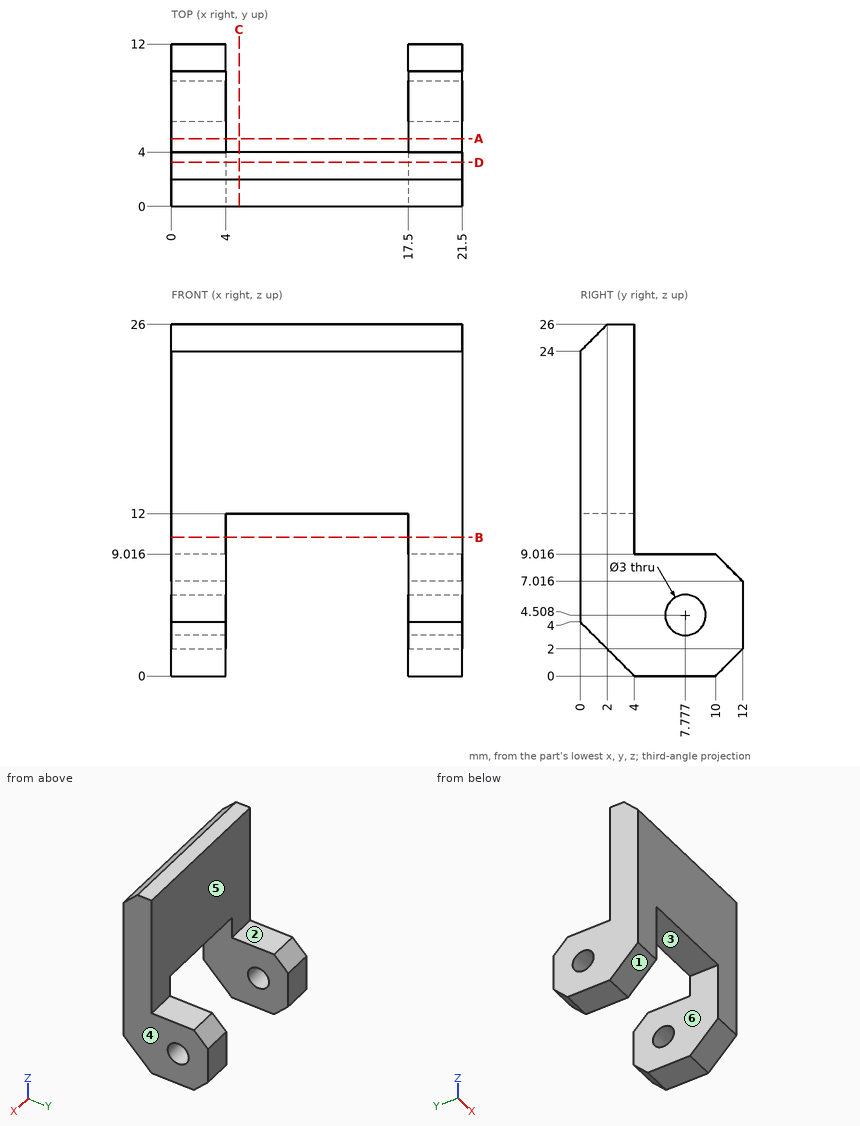
Check sheet for the drawn part. Datum: minimum x, y, z corner. Units: mm. A direction names the side the tool comes from. Round coordinates to 2 decimals unless told otherwise and drop trailing zeros. Write each loop counter-clockwise with the first axis right and the second up, starting at its lowest first coordinate (ties: lowest second). Pieces come first, ordered by that corner, then holes. Notation, with made-up numbers: (33, 5) -> (88, 5) arc R11 cw to (88, 9) -> close; hole circle Ø2 at (-33, 85.25). An arc over 180 degrees is marked (long way). Write each question's results on one line, items separated by ' | '. Start each with the question number.
1. Cross-section at C-C (x = 5). Enter the section's corners in (y, z).
2. Set-up check for the marked faces 1 and 2: record each of +Z, -Z, +X, -X, +Y, -Y from which the full face is reachable in a straight line by a thin tool's end or side.
3. Cross-section at B-B (z = 10.25). Enter the section's corners in (x, y).
4. Cross-section at A-A (y = 5). Enter the section's corners in (x, z).
5. Draft check along X on the marked faces 3, 4, 5 and 6. Enter one of: +X half, -X half, draft (parallel to the pull), parting line (faces both ways), or undercut.
6. Cross-section at D-D (y = 3.25). Enter the section's corners in (x, z).
7. Material ranges on probe 1 along X at (y, z) = (8.75, 3); probe 2 along Y at (x, z) = (8.25, 18.25); probe 3 along Z at (x, y) = (13, 2.75), recorded low to high. Write a range as from..to.
8. Depth check by flat-ended pin: P1, Ø5, axis at y = 4.5, z = 14, coming from the +X side; P2, Ø3, axis at x = 14, y = 3, coming from the -Z side; P3, Ø2, axis at x = 19, y = 8, coming from the +Z side; P4, Ø8.5, axis at x = 9, z = 16.5, coming from the +Y side. Enter the tip coordinate at first touch or a pass-through.
Solutions:
1) outline: (0, 12) -> (4, 12) -> (4, 26) -> (2, 26) -> (0, 24) -> close
2) face 1: -Z, +X, -X, -Y | face 2: +Z, +X, -X, +Y
3) outline: (0, 0) -> (4, 0) -> (4, 4) -> (0, 4) -> close; (17.5, 0) -> (21.5, 0) -> (21.5, 4) -> (17.5, 4) -> close
4) outline: (0, 0) -> (4, 0) -> (4, 9.02) -> (0, 9.02) -> close; (17.5, 0) -> (21.5, 0) -> (21.5, 9.02) -> (17.5, 9.02) -> close
5) face 3: undercut | face 4: +X half | face 5: draft | face 6: undercut
6) outline: (0, 0.75) -> (4, 0.75) -> (4, 12) -> (17.5, 12) -> (17.5, 0.75) -> (21.5, 0.75) -> (21.5, 26) -> (0, 26) -> close
7) probe 1: x = 0..4, 17.5..21.5 | probe 2: y = 0..4 | probe 3: z = 12..26
8) P1: stops at x = 21.5 | P2: stops at z = 12 | P3: stops at z = 9.02 | P4: stops at y = 4
